```python
from build123d import *

# Parameters (mm, degrees)
F0_W      = 42
F0_H      = 42
F1_DEPTH  = 8
F3_DEPTH  = 22
F4_W      = 42
F4_H      = 42
F5_DEPTH  = 9
F6_R      = 11
F6_R_2    = 4.5
F7_DEPTH  = 2
F8_R      = 2.5
F9_DEPTH  = 22
F11_DEPTH = 15
F12_R     = 1.5
F13_DEPTH = 4
F14_SIZE  = 4


with BuildPart() as f1:
    # F0 (on Front) → F1 (new body)
    with BuildSketch(Plane.XZ):
        with Locations((21, 21)):
            Rectangle(F0_W, F0_H)
    extrude(amount=F1_DEPTH)

    # F2 (on face) → F3 (join)
    with BuildSketch(Plane(origin=(0, 0, 0), x_dir=(-1, 0, 0), z_dir=(0, 1, 0))):
        with BuildLine():
            Line((0, 8), (0, 21))
            Line((0, 21), (0, 34))
            ThreePointArc((0, 34), (-2.3431457505, 39.6568542495), (-8, 42))
            Line((-8, 42), (-21, 42))
            Line((-21, 42), (-34, 42))
            ThreePointArc((-34, 42), (-39.6568542495, 39.6568542495), (-42, 34))
            Line((-42, 34), (-42, 21))
            Line((-42, 21), (-42, 8))
            ThreePointArc((-42, 8), (-39.6568542495, 2.3431457505), (-34, 0))
            Line((-34, 0), (-21, 0))
            Line((-21, 0), (-8, 0))
            ThreePointArc((-8, 0), (-2.3431457505, 2.3431457505), (0, 8))
        make_face()
    extrude(amount=F3_DEPTH)

    # F4 (on face) → F5 (join)
    with BuildSketch(Plane(origin=(0, 22, 0), x_dir=(-1, 0, 0), z_dir=(0, 1, 0))):
        with Locations((-21, 21)):
            Rectangle(F4_W, F4_H)
    extrude(amount=F5_DEPTH)

    # F6 (on face) → F7 (join)
    with BuildSketch(Plane.XZ.offset(8)):
        with Locations((21, 21)):
            Circle(F6_R)
        with Locations((21, 21)):
            Circle(F6_R_2, mode=Mode.SUBTRACT)
    extrude(amount=F7_DEPTH)

    # F8 (on face) → F9 (join)
    with BuildSketch(Plane.XZ.offset(8)):
        with Locations((21, 21)):
            Circle(F8_R)
    extrude(amount=F9_DEPTH)

    # F10 (on face) → F11 (cut)
    with BuildSketch(Plane.XZ.offset(30)):
        with BuildLine():
            Line((19.5, 19), (19.5, 23))
            ThreePointArc((19.5, 23), (18.7639320225, 22.1180339887), (18.5, 21))
            ThreePointArc((18.5, 21), (18.7639320225, 19.8819660113), (19.5, 19))
        make_face()
    extrude(amount=-F11_DEPTH, mode=Mode.SUBTRACT)

    # F12 (on face) → F13 (cut)
    with BuildSketch(Plane.XZ.offset(8)):
        with Locations((5.5, 5.5)):
            Circle(F12_R)
        with Locations((5.5, 36.5)):
            Circle(F12_R)
        with Locations((36.5, 36.5)):
            Circle(F12_R)
        with Locations((36.5, 5.5)):
            Circle(F12_R)
    extrude(amount=-F13_DEPTH, mode=Mode.SUBTRACT)

    # F14
    f14_edges = [f1.edges().sort_by_distance(p)[0] for p in [
        (0, -4, 42),
        (0, 26.5, 42),
        (42, -4, 42),
        (42, 26.5, 42),
        (42, 26.5, 0),
        (42, -4, 0),
        (0, -4, 0),
        (0, 26.5, 0),
    ]]
    chamfer(f14_edges, length=F14_SIZE)


solid = f1.part
```
Design review of the part built by this model. Coordinates are the model's own, in mm. A direction names the side the tool comes from. Give positions to 0.01 mm unless a question says otherwise; leave off trailing zeros. Loops run counter-clockwise (first coordinate to the right, second up) from the corner with the lowest first, then second, coordinate; pieces in that order, holes last. Notation, with made-up numbers: (54.5, 0) -> (113.5, 0) arc R8 cw to (113.5, 11) -> close; hole circle Ø7 at (-38.5, 51). An arc over 180 degrees is marked (long way). One line per item, written item: value.
Q1. We need section C-C on x = 21. Give the boundary of the cut face in (y, z).
Numbers:
outline: (-30, 18.5) -> (-8, 18.5) -> (-8, 16.5) -> (-10, 16.5) -> (-10, 10) -> (-8, 10) -> (-8, 0) -> (31, 0) -> (31, 42) -> (-8, 42) -> (-8, 32) -> (-10, 32) -> (-10, 25.5) -> (-8, 25.5) -> (-8, 23.5) -> (-30, 23.5) -> close
Q2. We need section D-D on y = -1.5. Give the boundary of the cut face in (x, z).
Numbers:
outline: (0, 4) -> (4, 0) -> (38, 0) -> (42, 4) -> (42, 38) -> (38, 42) -> (4, 42) -> (0, 38) -> close
Q3. We need section B-B on z = 21. Give the boundary of the cut face in (x, y), and give its area (3 significant figures).
Numbers:
outline: (0, -8) -> (10, -8) -> (10, -10) -> (16.5, -10) -> (16.5, -8) -> (18.5, -8) -> (18.5, -15) -> (19.5, -15) -> (19.5, -30) -> (23.5, -30) -> (23.5, -8) -> (25.5, -8) -> (25.5, -10) -> (32, -10) -> (32, -8) -> (42, -8) -> (42, 31) -> (0, 31) -> close
area: 1,760 mm^2
Q4. Machinability: for faces 1 (the cylindrical face through (23.31, -18.85, 20.04)), 2 (the flat face through (2.2, 22, 2.2)), 3 (the flat face through (39.8, 0, 2.2)), 4 (the flat face through (21, -30, 21)), which of the approach directions +Z, -Z, +X, -X, +Y, -Y give a long, thin tool a straight path to every point of the face, cutting with its end or side? Answer none if there is none.
Numbers:
face 1: -Y
face 2: -Z, -X
face 3: -Z, +X
face 4: +Z, -Z, +X, -X, -Y
Q5. Draft analysis for pull direction X (two halves, no side actions). For faces 5 (the cylindrical face through (35.3, -6, 4.6)), 6 (the flat face through (30, -8, 12)), 7 (the cylindrical face through (2.406, 10.846, 2.281)), state which applies: pulls with the +X half, pulls with the -X half, needs draft (parallel to the pull), parting line crosses it, or undercut.
Numbers:
face 5: undercut
face 6: needs draft
face 7: pulls with the -X half
Q6. For pin 1 Ø2.5 at (x, z) = (5.5, 5.5) entering from -Y; pin 2 Ø2.5 at (x, z) = (5.5, 37.5) entering from -Y; pin 3 Ø0.8 at (x, z) = (19, 22) entering from -Y; pin 4 Ø10 at (x, y) = (35, -19.5) entering from +Z, all flat-tipped, find the tip position at first contact; note any pin that passes through.
Numbers:
pin 1: stops at y = -4
pin 2: stops at y = -8
pin 3: stops at y = -15
pin 4: passes through
Q7. For L1, parallel to Z at x = 36.5, y = -5.3; L2, parallel to Z at x = 35.5, y = -7; L3, parallel to Y at x = 35, z = 29, list the stretches that pass through material, from the lowest coordinate up.
Numbers:
L1: z = 0 to 4, 7 to 35, 38 to 42
L2: z = 0 to 4.38, 6.62 to 35.38, 37.62 to 42
L3: y = -8 to 31
Q8. We need section A-A on y = 12. Give the boundary of the cut face in (x, z).
Numbers:
outline: (0, 8) arc R8 ccw to (8, 0) -> (34, 0) arc R8 ccw to (42, 8) -> (42, 34) arc R8 ccw to (34, 42) -> (8, 42) arc R8 ccw to (0, 34) -> close
